Geometry: see drawing. Coordinates: mm, zero at the bounding-box minimum. A direction names the side the tool comes from. Give positions to 0.01 mm unless a question says otherwise; leave off trailing zeros. Write each loop counter-clockwise with the first axis right and the second up, starting at its lowest first coordinate (ties: lowest second). Pieces come first, ordered by that corner, then holes.
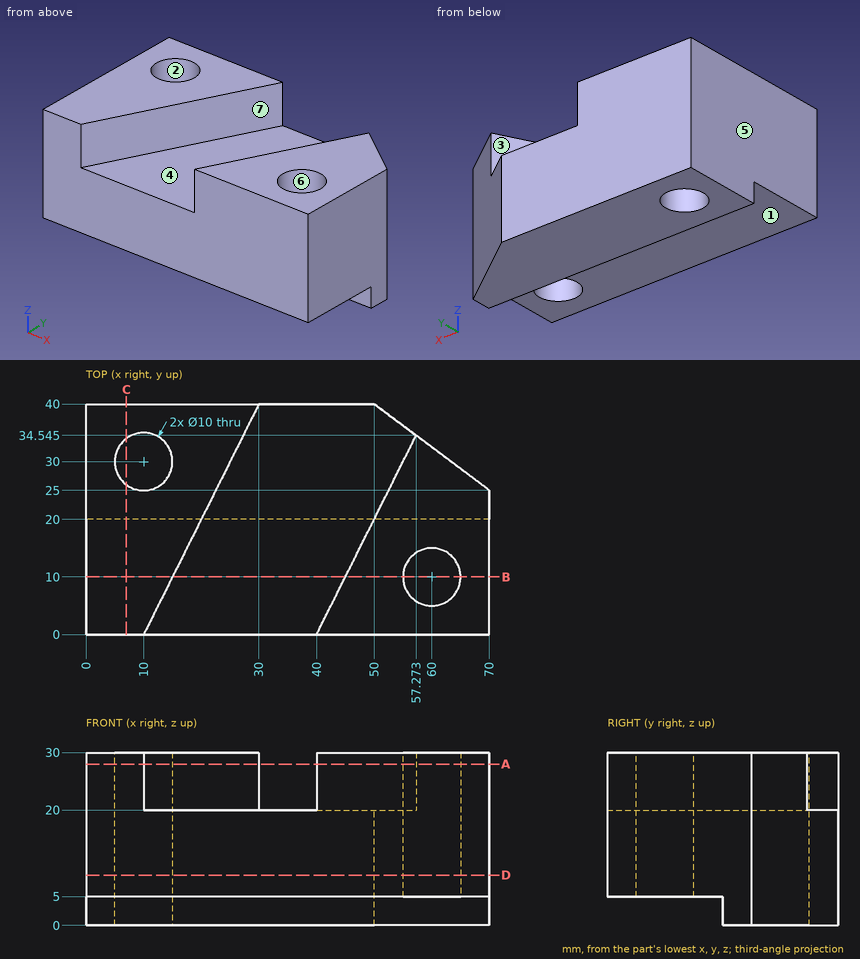
1. Pin query (flat end, axial travel): P1, Ø12, axis at x = 30, y = 18, coming from the +Z side; P2, Ø1.5, axis at x = 25.5, z = 3, coming from the -Y side; P3, Ø10, axis at x = 33.5, y = 14, coming from the -Z side. Return the tip coordinate at first contact, or that it passes through.
2. Pull-direction query (Y, two-part tool) for the marked faces 5, 6 and 7; classes: pulls with the +Y half, pulls with the -Y half, needs draft (parallel to the pull), parting line crosses it, or undercut.
3. Section query C-C (x = 7). Return loops of the section in (y, z).
4. Section query B-B (y = 10). Return loops of the section in (x, z), plus the area to 3 significant figures.
5. Section query A-A (z = 28). Return loops of the section in (x, y) (1 decimal).
6. Section query D-D (z = 8.75). Return loops of the section in (x, y).
7. Line query: probe 1 along Y at (x, z) = (10, 23.75); probe 2 along Z at (x, y) = (48.5, 12.5); probe 3 along Y at (x, z) = (64.5, 22.75) (1 decimal). Output: solid intervals per line, ascending.
8. Access query for the marked faces 1, 2, 3 and 4. Directions: +Z, -Z, +X, -X, +Y, -Y. A direction counts if a zero-diameter tool reaches every point of the face in a straight line with its end or side. Return the directions, or none.
The answers:
1. P1: stops at z = 20
1. P2: stops at y = 20
1. P3: stops at z = 5
2. face 5: needs draft
2. face 6: undercut
2. face 7: pulls with the -Y half
3. outline: (0, 5) - (20, 5) - (20, 0) - (26, 0) - (26, 30) - (0, 30) - close; (34, 0) - (40, 0) - (40, 30) - (34, 30) - close
4. outline: (0, 5) - (55, 5) - (55, 30) - (45, 30) - (45, 20) - (15, 20) - (15, 30) - (0, 30) - close; (65, 5) - (70, 5) - (70, 30) - (65, 30) - close
4. area: 1,200 mm2
5. outline: (0, 0) - (10, 0) - (30, 40) - (0, 40) - close; (40, 0) - (70, 0) - (70, 25) - (57.3, 34.5) - close; hole circle Ø10 at (10, 30); hole circle Ø10 at (60, 10)
6. outline: (0, 0) - (70, 0) - (70, 25) - (50, 40) - (0, 40) - close; hole circle Ø10 at (10, 30); hole circle Ø10 at (60, 10)
7. probe 1: y = 0 to 25, 35 to 40
7. probe 2: z = 5 to 30
7. probe 3: y = 0 to 7.8, 12.2 to 29.1
8. face 1: -Z, +X, -X, -Y
8. face 2: +Z, -Z
8. face 3: +Z, +Y
8. face 4: +Z
